Answer from the drawing. Dimensions are ordinates in mm from the lowest x, y and z of the part. Coordinates: 2 decimals unless noted, no trailing zeros. Loops run counter-clockwise (first coordinate to the right, second up) from the corner with the lowest first, then second, coordinate; pieces in that order, holes last. Notation, with made-up numbers: M -36,15 L 20,15 A16 ccw 20,30 Z; hole C 5,10.25 d7. An arc over 180 degrees is marked long. One line per item, written item: value. Start each with the question number.
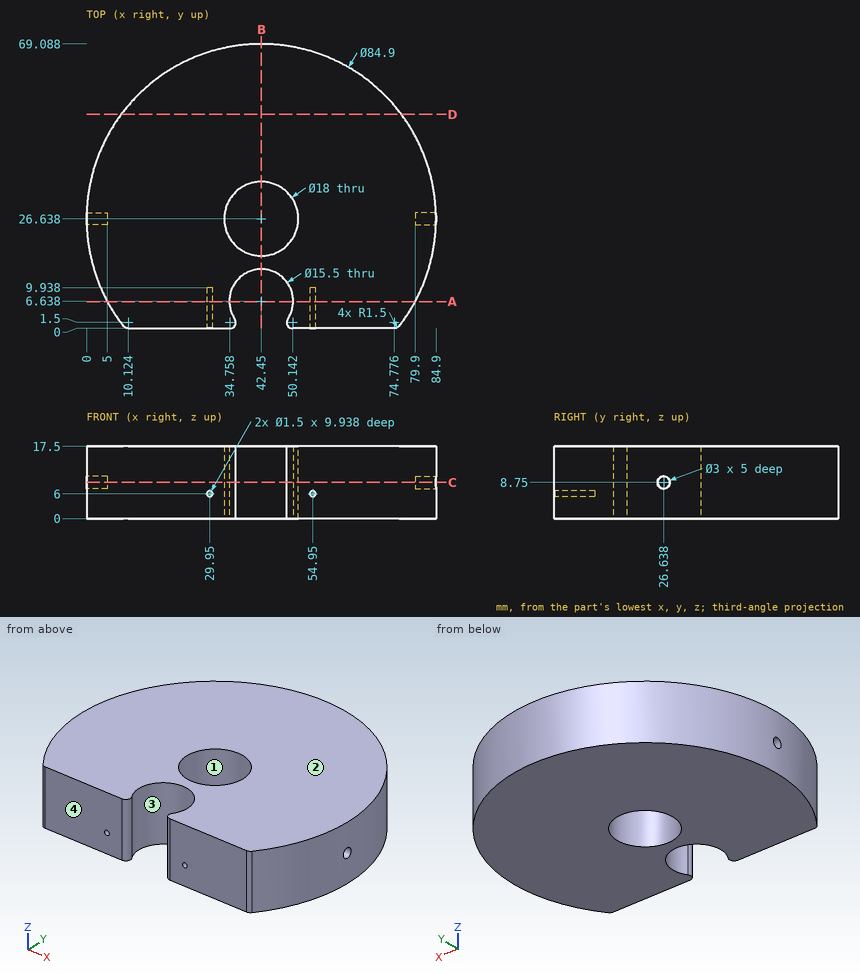
1) Section D-D (y = 52) is taken. Determine the outline of the cut face in (x, z).
2) For a pull along Y with two mould halves and no side action, classify the marked faces 1, 2, 3 and 4 as released by +Y, released by -Y, zero draft, split by the parting line, or undercut.
3) Consider line 1 along Z through (x, y) = (29.95, 6.75); line 2 along X through (y, z) = (4, 2.75); line 3 along X through (y, z) = (19.5, 7) (1 decimal). Determine where each line is inside the solid, lowest interval first.
4) Section C-C (z = 8.75) is taken. Determine the outline of the cut face in (x, y), then the cut area to 3 significant figures.
5) Section B-B (x = 42.45) is taken. Determine the outline of the cut face in (y, z).
6) Flat-ended cylindrical pins translate along their axes: pin 1 (4 mm diameter, centred on y = 26.64, z = 8.75, fed in from -X); pin 2 (3 mm diameter, centred on y = 22, z = 11, fed in from -X); pin 3 (2 mm diameter, centred on y = 48, z = 8, fed in from +X); pin 4 (2.5 mm diameter, centred on y = 26.64, z = 8.75, fed in from +X). Find the tip coordinate at first contact, or state that the pin passes through.
7) Section A-A (y = 6.5) is taken. Determine the outline of the cut face in (x, z).
Results found:
1. outline: M 8.41,0 L 76.49,0 L 76.49,17.5 L 8.41,17.5 Z
2. face 1: undercut
2. face 2: zero draft
2. face 3: undercut
2. face 4: released by -Y
3. line 1: z = 0 to 5.25, 6.75 to 17.5
3. line 2: x = 6.54 to 35.16, 49.74 to 78.36
3. line 3: x = 0.6 to 37, 47.9 to 84.3
4. outline: M 0.03,25.14 A42.45 ccw 8.94,0.58 A1.5 ccw 10.12,0 L 34.76,0 A1.5 ccw 36.01,2.33 A7.75 cw long 48.89,2.33 A1.5 ccw 50.14,0 L 74.78,0 A1.5 ccw 75.96,0.58 A42.45 ccw 84.87,25.14 L 79.9,25.14 L 79.9,28.14 L 84.87,28.14 A42.45 ccw 0.03,28.14 L 5,28.14 L 5,25.14 Z; hole C 42.45,26.64 d18
4. area: 4,460 mm²
5. outline: M 14.39,0 L 17.64,0 L 17.64,17.5 L 14.39,17.5 Z; M 35.64,0 L 69.09,0 L 69.09,17.5 L 35.64,17.5 Z
6. pin 1: stops at x = 0
6. pin 2: stops at x = 0.12
6. pin 3: stops at x = 79.7
6. pin 4: stops at x = 79.9
7. outline: M 5.08,0 L 34.7,0 L 34.7,17.5 L 5.08,17.5 Z; M 50.2,0 L 79.82,0 L 79.82,17.5 L 50.2,17.5 Z; hole C 29.95,6 d1.5; hole C 54.95,6 d1.5
